Autodesk Fusion 360 part; units mm, degrees
sketch "Sketch1" plane through (0, 0, 0) normal (0, 0, 1) x (1, 0, 0) in component "esp32-c3-devkitm-1"
  line L0 (14.6, 39.4) -> (-14.6, 39.4)
  line L1 (-14.6, 39.4) -> (-14.6, 0)
  line L2 (-14.6, 0) -> (14.6, 0)
  line L3 (14.6, 0) -> (14.6, 39.4)
  line L4 (14.6, 39.4) -> (-14.6, 0) construction
  line L5 (-14.6, 39.4) -> (14.6, 0) construction
  line L6 (0, 1.75) -> (0, 22.5)
  line L7 (1.75, 0) -> (22.5, 0)
  line L8 (6.6, 39.4) -> (-6.6, 39.4)
  line L9 (-6.6, 39.4) -> (-6.6, 29.4)
  line L10 (-6.6, 29.4) -> (6.6, 29.4)
  line L11 (6.6, 29.4) -> (6.6, 39.4)
  line L12 (6.6, 39.4) -> (-6.6, 29.4) construction
  line L13 (-6.6, 39.4) -> (6.6, 29.4) construction
  line L14 (6.6, 45) -> (-6.6, 45)
  line L15 (-6.6, 45) -> (-6.6, 39.4)
  line L16 (-6.6, 39.4) -> (6.6, 39.4)
  line L17 (6.6, 39.4) -> (6.6, 45)
  line L18 (6.6, 45) -> (-6.6, 39.4) construction
  line L19 (-6.6, 45) -> (6.6, 39.4) construction
  line L20 (-2.15, 7.35) -> (-11.1, 7.35)
  line L21 (-11.1, 7.35) -> (-11.1, 0)
  line L22 (-11.1, 0) -> (-2.15, 0)
  line L23 (-2.15, 0) -> (-2.15, 7.35)
  line L24 (-2.15, 7.35) -> (-11.1, 0) construction
  line L25 (-11.1, 7.35) -> (-2.15, 0) construction
  line L26 (11.1, 7.35) -> (2.15, 7.35)
  line L27 (2.15, 7.35) -> (2.15, 0)
  line L28 (2.15, 0) -> (11.1, 0)
  line L29 (11.1, 0) -> (11.1, 7.35)
  line L30 (11.1, 7.35) -> (2.15, 0) construction
  line L31 (2.15, 7.35) -> (11.1, 0) construction
  line L32 (2.5, 17.7) -> (-2.5, 17.7)
  line L33 (-2.5, 17.7) -> (-2.5, 12.7)
  line L34 (-2.5, 12.7) -> (2.5, 12.7)
  line L35 (2.5, 12.7) -> (2.5, 17.7)
  line L36 (2.5, 17.7) -> (-2.5, 12.7) construction
  line L37 (-2.5, 17.7) -> (2.5, 12.7) construction
  line L38 (9.6, 26.75) -> (4.6, 26.75)
  line L39 (4.6, 26.75) -> (4.6, 23.75)
  line L40 (4.6, 23.75) -> (9.6, 23.75)
  line L41 (9.6, 23.75) -> (9.6, 26.75)
  line L42 (9.6, 26.75) -> (4.6, 23.75) construction
  line L43 (4.6, 26.75) -> (9.6, 23.75) construction
  line L44 (9.6, 22.55) -> (4.6, 22.55)
  line L45 (4.6, 22.55) -> (4.6, 19.55)
  line L46 (4.6, 19.55) -> (9.6, 19.55)
  line L47 (9.6, 19.55) -> (9.6, 22.55)
  line L48 (9.6, 22.55) -> (4.6, 19.55) construction
  line L49 (4.6, 22.55) -> (9.6, 19.55) construction
  circle A0 centre (7.1, 25.25) radius 0.9
  circle A1 centre (7.1, 21.05) radius 0.9
  circle A2 centre (12.95, 37.025) radius 0.5
  circle A3 centre (-12.95, 37.025) radius 0.5
  circle A4 centre (12.95, 34.485) radius 0.5
  circle A5 centre (-12.95, 34.485) radius 0.5
  circle A6 centre (12.95, 31.945) radius 0.5
  circle A7 centre (-12.95, 31.945) radius 0.5
  circle A8 centre (12.95, 29.405) radius 0.5
  circle A9 centre (-12.95, 29.405) radius 0.5
  circle A10 centre (12.95, 26.865) radius 0.5
  circle A11 centre (-12.95, 26.865) radius 0.5
  circle A12 centre (12.95, 24.325) radius 0.5
  circle A13 centre (-12.95, 24.325) radius 0.5
  circle A14 centre (12.95, 21.785) radius 0.5
  circle A15 centre (-12.95, 21.785) radius 0.5
  circle A16 centre (12.95, 19.245) radius 0.5
  circle A17 centre (-12.95, 19.245) radius 0.5
  circle A18 centre (12.95, 16.705) radius 0.5
  circle A19 centre (-12.95, 16.705) radius 0.5
  circle A20 centre (12.95, 14.165) radius 0.5
  circle A21 centre (-12.95, 14.165) radius 0.5
  circle A22 centre (12.95, 11.625) radius 0.5
  circle A23 centre (-12.95, 11.625) radius 0.5
  circle A24 centre (12.95, 9.085) radius 0.5
  circle A25 centre (-12.95, 9.085) radius 0.5
  circle A26 centre (12.95, 6.545) radius 0.5
  circle A27 centre (-12.95, 6.545) radius 0.5
  circle A28 centre (12.95, 4.005) radius 0.5
  circle A29 centre (-12.95, 4.005) radius 0.5
  circle A30 centre (12.95, 1.465) radius 0.5
  circle A31 centre (-12.95, 1.465) radius 0.5
  point P0 (0, 19.7)
  point P1 (0, 34.4)
  point P2 (0, 42.2)
  point P3 (-6.625, 3.675)
  point P4 (6.625, 3.675)
  point P5 (0, 15.2)
  point P6 (7.1, 25.25)
  point P7 (7.1, 21.05)
  dimension "d22" = 29.2
  dimension "d23" = 39.4
  dimension "d24" = 13.2
  dimension "d25" = 10
  dimension "d26" = 13.2
  dimension "d27" = 5.6
  dimension "d28" = 8.95
  dimension "d29" = 7.35
  dimension "d31" = 3.5
  dimension "d32" = 8.95
  dimension "d33" = 7.35
  dimension "d34" = 3.5
  dimension "d35" = 5
  dimension "d36" = 5
  dimension "d37" = 17.7
  dimension "d41" = 5
  dimension "d42" = 3
  dimension "d43" = 10
  dimension "d44" = 12.65
  dimension "d45" = 5
  dimension "d46" = 3
  dimension "d47" = 1.2
  dimension "d48" = 1.8
  dimension "d49" = 1.8
  dimension "d95" = 2.375
  dimension "d96" = 1.65
  dimension "d99" = -25.9
  dimension "d105" = 1
extrude "Extrude1" add sketch "Sketch1" along normal blind 1.6 contours L0 L1 L2 L3 L7 L9 L10 L11 L20 L21 L23 L26 L27 L29 | A2 | A3 | A4 | A5 | A6 | A7 | A8 | A9 | A10 | A11 | A12 | A13 | A14 | A15 | A16 | A17 | A18 | A19 | A20 | A21 | A22 | A23 | A24 | A25 | A26 | A27 | A28 | A29 | A30 | A31 in component "esp32-c3-devkitm-1"
extrude "Extrude2" add sketch "Sketch1" along normal blind 4.9 contours L2 L7 L26 L27 L28 L29 | L2 L20 L21 L22 L23 in component "esp32-c3-devkitm-1"
extrude "Extrude3" add sketch "Sketch1" along normal blind 4.1 contours L0 L8 L9 L10 L11 L16 in component "esp32-c3-devkitm-1"
extrude "Extrude4" add sketch "Sketch1" along normal blind 3.15 contours L6 L32 L33 L34 | L6 L32 L34 L35 in component "esp32-c3-devkitm-1"
extrude "Extrude5" add sketch "Sketch1" along normal blind 3.15 contours L38 L39 L40 L41 | L44 L45 L46 L47 in component "esp32-c3-devkitm-1"
extrude "Extrude6" add sketch "Sketch1" along normal blind 3.65 contours A0 | A1 in component "esp32-c3-devkitm-1"
extrude "Extrude7" add sketch "Sketch1" along normal blind 0.8 from surface at 1.6 contours L0 L8 L14 L15 L16 L17 in component "esp32-c3-devkitm-1"
fillet "Fillet1" radius 1.2 4 edges at (-11.1, 3.675, 4.9) (-2.15, 3.675, 4.9) (2.15, 3.675, 4.9) (11.1, 3.675, 4.9) in component "esp32-c3-devkitm-1"
sketch "Sketch2" plane through (0, 0, 0) normal (0, -1, 0) x (1, 0, 0) in component "esp32-c3-devkitm-1"
  arc A0 (11.1, 3.7) -> (9.9, 4.9) centre (9.9, 3.7) ccw
  line L0 (9.9, 4.9) -> (3.35, 4.9)
  arc A1 (3.35, 4.9) -> (2.15, 3.7) centre (3.35, 3.7) ccw
  line L1 (2.15, 3.7) -> (2.15, 1.6)
  line L2 (2.15, 1.6) -> (-2.15, 1.6)
  line L3 (-2.15, 1.6) -> (-2.15, 3.7)
  arc A2 (-2.15, 3.7) -> (-3.35, 4.9) centre (-3.35, 3.7) ccw
  line L4 (-3.35, 4.9) -> (-9.9, 4.9)
  arc A3 (-9.9, 4.9) -> (-11.1, 3.7) centre (-9.9, 3.7) ccw
  line L5 (-11.1, 3.7) -> (-11.1, 1.6)
  line L6 (-11.1, 1.6) -> (-14.6, 1.6)
  line L7 (-14.6, 1.6) -> (-14.6, 0)
  line L8 (-14.6, 0) -> (14.6, 0)
  line L9 (14.6, 0) -> (14.6, 1.6)
  line L10 (14.6, 1.6) -> (11.1, 1.6)
  line L11 (11.1, 1.6) -> (11.1, 3.7)
  line L12 (-9.45, 4.6) -> (-3.8, 4.6)
  line L13 (-9.45, 1.9) -> (-3.8, 1.9)
  arc A4 (-9.45, 4.6) -> (-9.45, 1.9) centre (-9.45, 3.25) ccw
  arc A5 (-3.8, 1.9) -> (-3.8, 4.6) centre (-3.8, 3.25) ccw
  arc A6 (9.45, 1.9) -> (9.45, 4.6) centre (9.45, 3.25) ccw
  line L14 (3.8, 1.9) -> (9.45, 1.9)
  arc A7 (3.8, 4.6) -> (3.8, 1.9) centre (3.8, 3.25) ccw
  line L15 (3.8, 4.6) -> (9.45, 4.6)
  dimension "d80" = 0.3
  dimension "d81" = 1.65
  dimension "d83" = 0.3
  dimension "d86" = 0.3
  dimension "d87" = 1.65
  dimension "d88" = 1.65
  dimension "d89" = 1.65
  dimension "d90" = 1.65
  dimension "d91" = 0.3
  dimension "d92" = 1.65
  dimension "d93" = 1.65
  dimension "d94" = 1.65
extrude "Extrude8" cut sketch "Sketch2" against normal blind 7 contours L12 L13 A4 A5 | A6 L14 A7 L15 in component "esp32-c3-devkitm-1"
hole "Hole2" at (12.95, 37.025, 0) at (12.95, 34.485, 0) at (12.95, 31.945, 0) at (12.95, 29.405, 0) at (12.95, 26.865, 0) at (12.95, 24.325, 0) at (0, 0, 0) at (12.95, 19.245, 0) at (12.95, 16.705, 0) at (12.95, 14.165, 0) at (12.95, 11.625, 0) at (12.95, 9.085, 0) at (12.95, 6.545, 0) at (12.95, 4.005, 0) at (12.95, 1.465, 0) at (-12.95, 1.465, 0) at (-12.95, 4.005, 0) at (-12.95, 6.545, 0) at (-12.95, 9.085, 0) at (-12.95, 11.625, 0) at (-12.95, 14.165, 0) at (-12.95, 16.705, 0) at (-12.95, 19.245, 0) at (0, 0, 0) at (-12.95, 24.325, 0) at (-12.95, 26.865, 0) at (-12.95, 29.405, 0) at (-12.95, 31.945, 0) at (-12.95, 34.485, 0) at (-12.95, 37.025, 0) direction (0, 0, 1) diameter 0.75 depth 11 tip angle 118 in component "esp32-c3-devkitm-1"
component "esp32-c3-devkitm-1" placed x (1, 0, 0) y (0, 1, 0) z (0, 0, 1) at (0, 0, 0)
equation "pcb_thickness = 1.6 mm"
equation "module_height = 2.5 mm"
equation "usb_height = 3.3 mm"
equation "button_modue_height = 1.55 mm"
equation "button_height = 0.5 mm"
equation "button_diameter = 1.8 mm"
equation "led_height = 1.55 mm"
equation "led_width_length = 5 mm"
equation "usb_width = 8.95 mm"
equation "usb_length = 7.35 mm"
equation "board_length = 39.4 mm"
equation "board_width = 29.2 mm"
equation "overall_length = 45 mm"
equation "module_width = 13.2 mm"
equation "module_length = 10 mm"
equation "button_module_width = 3 mm"
equation "button_module_length = 5 mm"
equation "pin_spacing = 2.54 mm"
equation "d22 = board_width"
equation "d23 = board_length"
equation "d24 = module_width"
equation "d25 = module_length"
equation "d26 = module_width"
equation "d27 = overall_length - board_length"
equation "d28 = usb_width"
equation "d29 = usb_length"
equation "d32 = usb_width"
equation "d33 = usb_length"
equation "d35 = led_width_length"
equation "d36 = led_width_length"
equation "d41 = button_module_length"
equation "d42 = button_module_width"
equation "d44 = 15.65 mm - button_module_width"
equation "d45 = button_module_length"
equation "d46 = button_module_width"
equation "d48 = button_diameter"
equation "d49 = button_diameter"
equation "d50 = pcb_thickness"
equation "d52 = pcb_thickness + usb_height"
equation "d54 = pcb_thickness + module_height"
equation "d56 = pcb_thickness + led_height"
equation "d58 = pcb_thickness + button_modue_height"
equation "d60 = pcb_thickness + button_modue_height + button_height"
equation "d62 = pcb_thickness"
equation "d99 = -( board_width - 1.65 mm - 1.65 mm )"
equation "pin_diameter = 1 mm"
equation "d105 = pin_diameter"
equation "tolerance_loose = 0.508 mm"
equation "tolerance_tight = 0.127 mm"
equation "tolerance_normal = 0.254 mm"
equation "sma_base_plate_widthy = 6.55 mm"
equation "antenna_board_thickness = 3.225 mm"
equation "sma_base_plate_thickness = 1.65 mm"
equation "antenna_header_width_offset = 5.25 mm"
equation "antenna_header_length_offset = 1.3 mm"
equation "sma_base_plate_vertical_offset = 1 mm"
equation "antenna_board_length_Copy = 33.3 mm"
equation "antenna_board_width = 18 mm"
equation "sma_width_offset = 9 mm"
equation "sma_diameter = 6.26 mm"
equation "antenna_sma_wall_thickness = 3.15 mm"
For this review, take the finished solid that the model builds, in its own axes (mm). A direction names the side the tool comes from. Coordinates: 2 decimals unless noted, no trailing zeros. Order: outer loops, then holes, each group sorted by start corner. A loop starts at its lowest first (then second) coordinate and runs counter-clockwise, first axis right, second up. Notation, with made-up numbers: (46, -25) - (102, -25) arc R28 ccw to (102, 13) - close; hole circle Ø10 at (14.5, -39). An arc over 180 degrees is marked (long way). Use one line per item in the form item = value.
Q1. For faces 4 (the flat face through (-7, 7.35, 3)), 5 (the flat face through (9.6, 25, 2)), 6 (the flat face through (0, 42, 2.4)), 7 (the flat face through (0, 42, 1.6)), 8 (the flat face through (-11.1, 4, 3)), list the 3-axis set-ups (+Z, -Z, +X, -X, +Y, -Y) from which the entire face can be reached by the end or side of a thin tool; tool diameter is ignored.
Checked values:
face_4 = +Z, +X, -X
face_5 = +Z, +X, +Y
face_6 = +Z, +X, -X, +Y
face_7 = -Z, +X, -X, +Y
face_8 = +Z, -X, +Y, -Y
Q2. Draft analysis for pull direction X (two halves, no side actions). For faces 1 (the flat face through (4.6, 21, 2)), 2 (the cylindrical face through (-10.8, 3.5, 3.3)), 3 (the flat face through (7, 19.55, 2)), state which applies: +X half, -X half, draft (parallel to the pull), parting line (faces both ways), or undercut.
Checked values:
face_1 = -X half
face_2 = undercut
face_3 = draft
Q3. Consider section A-A (y = 21.05). Give the boundary of the cut face in (x, z).
Checked values:
outline = (-14.6, 0) - (14.6, 0) - (14.6, 1.6) - (9.6, 1.6) - (9.6, 3.15) - (8, 3.15) - (8, 3.65) - (6.2, 3.65) - (6.2, 3.15) - (4.6, 3.15) - (4.6, 1.6) - (-14.6, 1.6) - close
Q4. For probe 1 along Z at (x, y) = (4.25, 3); probe 2 along Y at (x, z) = (3, 2.55); probe 3 along X at (y, z) = (19.5, 1.3), list the stretches that pass through material, from the lowest coordinate up. Write a range as from..to.
Checked values:
probe_1 = 0..1.9, 4.6..4.9
probe_2 = 7..7.35, 29.4..39.4
probe_3 = -14.6..-13.22, -12.68..12.68, 13.22..14.6
Q5. Consider section D-D (y = 15). Give the boundary of the cut face in (x, z).
Checked values:
outline = (-14.6, 0) - (14.6, 0) - (14.6, 1.6) - (2.5, 1.6) - (2.5, 3.15) - (-2.5, 3.15) - (-2.5, 1.6) - (-14.6, 1.6) - close
Q6. Consider section C-C (x = 1.5). Give the boundary of the cut face in (y, z), then the cut area to 3 significant figures.
Checked values:
outline = (0, 0) - (39.4, 0) - (39.4, 1.6) - (45, 1.6) - (45, 2.4) - (39.4, 2.4) - (39.4, 4.1) - (29.4, 4.1) - (29.4, 1.6) - (17.7, 1.6) - (17.7, 3.15) - (12.7, 3.15) - (12.7, 1.6) - (0, 1.6) - close
area = 100 mm2
Q7. For P1, Ø1.7, axis at y = 24.5, z = 2, coming from the +X side; P2, Ø0.5, axis at y = 25, z = 2, coming from the -X side; P3, Ø11, axis at x = -3, y = 34.5, coming from the +Z side; P4, Ø2, axis at x = -7, z = 3.5, coming from the -Y side, all flat-tipped, find the tip position at first contact; note any pin that passes through.
Checked values:
P1 = 14.6
P2 = 4.6
P3 = 4.1
P4 = 7
Q8. Consider section B-B (z = 0.9). Give the number of separate pieces and of enclosed holes in the cut face, then the cut area to 3 significant figures.
Checked values:
separate_pieces = 1
enclosed_holes = 28
area = 1,140 mm2
